Verification items for the finished model (mm, model axes). Round coordinates to 2 decimals unless told otherwise and drop trailing zeros. Write each loop counter-clockwise with the first axis right and the second up, starting at its lowest first coordinate (ties: lowest second). Pieces come first, ordered by that corner, then holes. Notation, with made-up numbers: M -4.75,54 L 29.25,54 A26 cw 29.25,76 Z; hole C 78,86 d1. An arc over 180 degrees is marked long. Use a Markdown table: item, result. Add a question column.
from build123d import *

# Parameters (mm, degrees)
CROQUIS1_W              = 8
CROQUIS1_H              = 8
SALIENTE_EXTRUIR1_DEPTH = 76
CROQUIS2_R              = 2.5
SALIENTE_EXTRUIR2_DEPTH = 5
SALIENTE_EXTRUIR3_START = 5
CROQUIS3_R              = 2.5
SALIENTE_EXTRUIR3_DEPTH = 5


with BuildPart() as part:
    # Croquis1 → Saliente-Extruir1 (new, symmetric)
    with BuildSketch(Plane.XY):
        Rectangle(CROQUIS1_W, CROQUIS1_H)
    extrude(amount=SALIENTE_EXTRUIR1_DEPTH, both=True)

    # Croquis2 → Saliente-Extruir2 (add)
    with BuildSketch(Plane.XY.offset(76)):
        with Locations(Location((0, 0, 0), (0, 0, 180))):
            Circle(CROQUIS2_R)
    extrude(amount=SALIENTE_EXTRUIR2_DEPTH)

    # Croquis3 → Saliente-Extruir3 (add)
    with BuildSketch(Plane(origin=(0, 0, -76), x_dir=(-1, 0, 0), z_dir=(0, 0, -1)).offset(SALIENTE_EXTRUIR3_START)):
        Circle(CROQUIS3_R)
    extrude(amount=-SALIENTE_EXTRUIR3_DEPTH)


solid = part.part
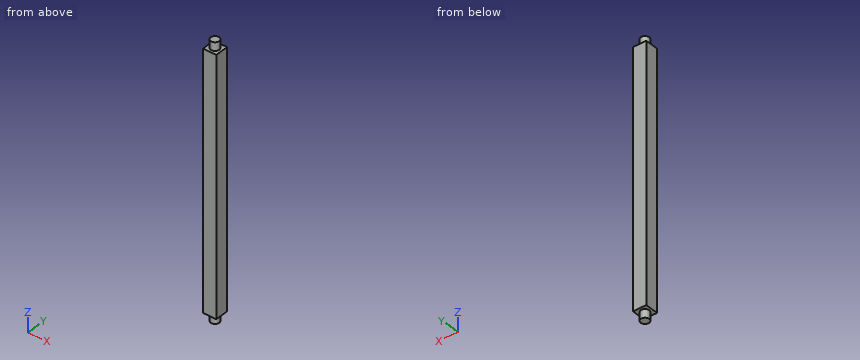
1. Scan line: line 1 along Z through (x, y) = (-2, 3). Record every from-to range of solid material in increasing order. Write a range as from..to.
2. Cross-section at A-A on x = 0. Enter the section's corners in (y, z), plus the area to 3 significant figures.
Answer:
| question | item | result |
|---|---|---|
| 1 | line 1 | z = -76..76 |
| 2 | outline | M -4,-76 L -2.5,-76 L -2.5,-81 L 2.5,-81 L 2.5,-76 L 4,-76 L 4,76 L 2.5,76 L 2.5,81 L -2.5,81 L -2.5,76 L -4,76 Z |
| 2 | area | 1,270 mm^2 |
